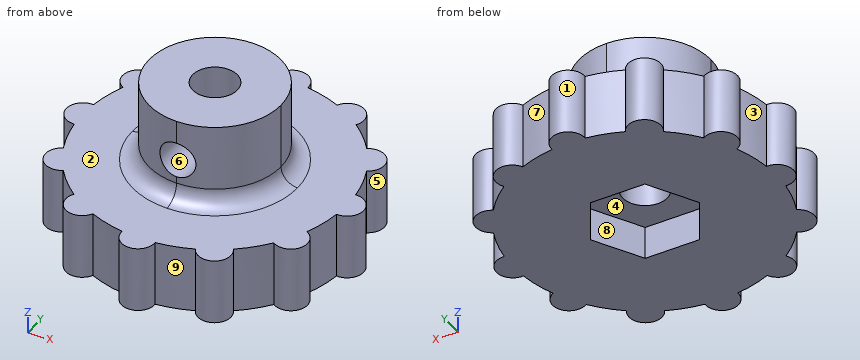
from build123d import *

# Parameters (mm, degrees)
F0_R         = 12.7
F1_DEPTH     = 6.35
F3_DEPTH     = 3.175
F4_W         = 12.7
F4_H         = 12.7
F5_DEPTH     = 7.9375
F7_DEPTH     = 6.35
F8_COUNT     = 12
F8_ANGLE     = 330
F9_R         = 2.15265
F10_DEPTH    = 11.1125
F11_R        = 1.7272
F12_REACH    = 25.5237593299
F13_T1_DEPTH = 7.9375
F14_R        = 1.5875


# Not quite as in the source:
# - a fillet or chamfer that OpenCascade refuses, or shapes differently, is made with other operations: its cross-section is extruded or revolved along the edge and cut away or added


with BuildPart() as f1:
    # F0 (on Top) → F1 (new body)
    with BuildSketch(Plane.XY):
        Circle(F0_R)
    extrude(amount=F1_DEPTH)

    # F2 (on face) → F3 (cut)
    with BuildSketch(Plane(origin=(0, 0, 0), x_dir=(1, 0, 0), z_dir=(0, 0, -1))):
        Polygon((2.6100007461, 4.5206539), (-2.6100007461, 4.5206539), (-5.2200014922, 0), (-2.6100007461, -4.5206539), (2.6100007461, -4.5206539), (5.2200014922, 0), align=None)
    extrude(amount=-F3_DEPTH, mode=Mode.SUBTRACT)

    # F4 (on face) → F5 (join)
    with BuildSketch(Plane.XY.offset(6.35)):
        Rectangle(F4_W, F4_H)
    extrude(amount=F5_DEPTH)

    # F6 (on face) → F7 (join, through all)
    with BuildSketch(Plane(origin=(0, 0, 0), x_dir=(1, 0, 0), z_dir=(0, 0, -1))):
        with BuildLine():
            ThreePointArc((-1.5843963802, 12.60078125), (0, 12.7), (1.5843963802, 12.60078125))
            ThreePointArc((1.5843963802, 12.60078125), (0, 14.2875), (-1.5843963802, 12.60078125))
        make_face()
    f7 = extrude(amount=-F7_DEPTH)

    # F8: F7 ×12 about axis
    f8_axis = Axis((0, 0, 0), (0, 0, -1))
    for i in range(1, F8_COUNT):
        add(f7.rotate(f8_axis, i * F8_ANGLE / (F8_COUNT - 1)))

    # F9 (on face) → F10 (cut, through all)
    with BuildSketch(Plane(origin=(0, 0, 3.175), x_dir=(1, 0, 0), z_dir=(0, 0, -1))):
        Circle(F9_R)
    extrude(amount=-F10_DEPTH, mode=Mode.SUBTRACT)

    f12_end = f1.faces().sort_by_distance((-2.15265, 0, 8.73125))[0]
    # F11 (on face) → F12 (cut, up to a face of the model that its end follows)
    with BuildSketch(Plane.XZ.offset(6.35)):
        with Locations((0, 10.31875)):
            Circle(F11_R)
    f12_long = extrude(amount=-F12_REACH, mode=Mode.PRIVATE)
    add(split(f12_long, bisect_by=f12_end, keep=Keep.ALL, mode=Mode.PRIVATE).solids().sort_by_distance((0, -6.35, 10.31875))[0], mode=Mode.SUBTRACT)

    # F13: fillet of radius 6.35 on 4 edges, made by hand

    # F13_s2 → F13_t1 (cut)
    with BuildSketch(Plane.XY.offset(6.35)):
        with BuildLine():
            ThreePointArc((0, -6.35), (-4.4901280605, -4.4901280605), (-6.35, 0))
            Line((-6.35, 0), (-6.477, 0))
            Line((-6.477, 0), (-6.477, -6.477))
            Line((-6.477, -6.477), (0, -6.477))
            Line((0, -6.477), (0, -6.35))
        make_face()
        with BuildLine():
            ThreePointArc((6.35, 0), (4.4901280605, -4.4901280605), (0, -6.35))
            Line((0, -6.35), (0, -6.477))
            Line((0, -6.477), (6.477, -6.477))
            Line((6.477, -6.477), (6.477, 0))
            Line((6.477, 0), (6.35, 0))
        make_face()
        with BuildLine():
            ThreePointArc((6.35, 0), (4.4901280605, 4.4901280605), (0, 6.35))
            Line((0, 6.35), (0, 6.477))
            Line((0, 6.477), (6.477, 6.477))
            Line((6.477, 6.477), (6.477, 0))
            Line((6.477, 0), (6.35, 0))
        make_face()
        with BuildLine():
            ThreePointArc((-6.35, 0), (-4.4901280605, 4.4901280605), (0, 6.35))
            Line((0, 6.35), (0, 6.477))
            Line((0, 6.477), (-6.477, 6.477))
            Line((-6.477, 6.477), (-6.477, 0))
            Line((-6.477, 0), (-6.35, 0))
        make_face()
    extrude(amount=F13_T1_DEPTH, mode=Mode.SUBTRACT)

    # F14
    f14_edges = [f1.edges().sort_by_distance(p)[0] for p in [
        (4.490128, 4.490128, 6.35),
    ]]
    fillet(f14_edges, radius=F14_R)


solid = f1.part
For this review, take the finished solid that the model builds, in its own axes (mm). Face numbers are marked on the shaded views. A direction names the side the tool comes from. Round coordinates to 2 decimals unless told otherwise and drop trailing zeros. Loops run counter-clockwise (first coordinate to the right, second up) from the corner with the lowest first, then second, coordinate; pieces in that order, holes last. Notation, with made-up numbers: (-29, -3) - (-6, -3) arc R16 cw to (-6, 24) - close; hole circle Ø3 at (-18, -9.5). An arc over 180 degrees is marked (long way). One line per item, written item: value. Start each with the question number.
Item 1: For L1, parallel to Z at x = 0, y = -2.75 (1 decimal); L2, parallel to Z at x = -12.5, y = 0.75; L3, parallel to Y at x = 0, z = 11.25, list the stretches that pass through material, from the lowest coordinate up.
Item 2: For the marked faces 5, 6, 7, 8 and 9, list the 3-axis set-ups (+Z, -Z, +X, -X, +Y, -Y) from which the entire face can be reached by the end or side of a thin tool; tool diameter is ignored.
Item 3: Take a section at C-C (x = 11.25). Give the boundary of the cut face in (y, z), plus the area to 3 significant figures.
Item 4: Take a section at B-B (z = 9.75). Give the boundary of the cut face in (x, y).
Item 5: Take a section at D-D (z = 12.5). Give the boundary of the cut face in (x, y).
Item 6: Clearance check with flat-ended pins moving along their axes: pin 1 Ø3 at (y, z) = (6, 3) entering from -X; pin 2 Ø5 at (x, y) = (7, 0) entering from +Z; pin 3 Ø4.5 at (x, z) = (0, 10.32) entering from -Y; pin 4 Ø1.6 at (x, z) = (-1, 1) entering from -Y. State where each tip first meets the part, or that it passes through.
Item 7: The part is to be moulded in two halves that separate along X. For the marked faces 1, 2, 3 and 4, say which applies: +X half, -X half, draft (parallel to the pull), parting line (faces both ways), or undercut.
Answer below:
1. L1: z = 3.2 to 8.6, 12 to 14.3
1. L2: z = 0 to 6.35
1. L3: y = 2.15 to 6.35
2. face 5: +Z, -Z
2. face 6: -Y
2. face 7: +Z, -Z, +Y
2. face 8: -Z
2. face 9: +Z, -Z, -Y
3. outline: (-7.92, 0) - (7.92, 0) - (7.92, 6.35) - (-7.92, 6.35) - close
3. area: 101 mm2
4. outline: (-1.63, -6.14) - (-1.63, -1.41) arc R2.15 cw (long way) to (1.63, -1.41) - (1.63, -6.14) arc R6.35 ccw (long way) to start
5. outline: circle Ø12.7 at (0, 0); hole circle Ø4.31 at (0, 0)
6. pin 1: stops at x = -12.59
6. pin 2: stops at z = 14.29
6. pin 3: stops at y = -6.35
6. pin 4: stops at y = -14.27
7. face 1: parting line
7. face 2: draft
7. face 3: -X half
7. face 4: undercut
